from build123d import *

# Parameters (mm, degrees)
SKETCH1_W           = 30
SKETCH1_H           = 30
SKETCH1_W_2         = 26
SKETCH1_H_2         = 26
BOSS_EXTRUDE1_DEPTH = 248
SKETCH2_R           = 12
SKETCH2_R_2         = 10
BOSS_EXTRUDE2_DEPTH = 5


with BuildPart() as part:
    # Sketch1 → Boss-Extrude1 (new body)
    with BuildSketch(Plane.XY):
        Rectangle(SKETCH1_W, SKETCH1_H)
        Rectangle(SKETCH1_W_2, SKETCH1_H_2, mode=Mode.SUBTRACT)
    extrude(amount=BOSS_EXTRUDE1_DEPTH)

    # Sketch2 → Boss-Extrude2 (add)
    # profile 1 of 2: a face of its own
    with BuildSketch(Plane(origin=(15, 0, 0), x_dir=(0, 0, -1), z_dir=(1, 0, 0))):
        with Locations(Location((-19.522331238, 0, 0), (0, 0, 180))):
            Circle(SKETCH2_R)
        with Locations((-19.522331238, 0)):
            Circle(SKETCH2_R_2, mode=Mode.SUBTRACT)
    # profile 2 of 2: a face of its own
    with BuildSketch(Plane(origin=(15, 0, 0), x_dir=(0, 0, -1), z_dir=(1, 0, 0))):
        with Locations(Location((-228.477668762, 0, 0), (0, 0, 180))):
            Circle(SKETCH2_R)
        with Locations(Location((-228.477668762, 0, 0), (0, 0, 180))):
            Circle(SKETCH2_R_2, mode=Mode.SUBTRACT)
    extrude(amount=BOSS_EXTRUDE2_DEPTH)


solid = part.part
Source: CAD feature listing. Evaluate the final solid. Frame: model axes, mm. A direction names the side the tool comes from. Give positions to 0.01 mm unless a question says otherwise; leave off trailing zeros. Write each loop counter-clockwise with the first axis right and the second up, starting at its lowest first coordinate (ties: lowest second). Pieces come first, ordered by that corner, then holes. Notation, with made-up numbers: M 15,78.25 L 74,78.25 A28 ccw 74,104.25 Z; hole C 85,41.5 d11. An arc over 180 degrees is marked long. Return JSON: item names as keys, results as strings. Group by question number.
1) Cut plane C-C, the plane z = 154.5. Output: boundary loops of the cut face in (x, y), plus the area to 3 significant figures.
2) Cut plane D-D, the plane z = 227. Output: boundary loops of the cut face in (x, y).
3) Pin query (flat end, axial travel): P1, Ø1.5, axis at y = -4, z = 118.5, coming from the +X side. Return the tip coordinate at first contact, or that it passes through.
4) Pull-direction query (Y, two-part tool) for faces 4 (the face through (-13, 0, 122)), 5 (the face through (15, 0, 122)), 6 (the face through (0, -15, 122)); classes: pulls with the +Y half, pulls with the -Y half, needs draft (parallel to the pull), parting line crosses it, or undercut.
5) Set-up query: faces 1 (the face through (15, 0, 228)), 2 (the face through (-14, 0, 248)), 3 (the face through (13, 0, 122)). Return all of +Z, -Z, +X, -X, +Y, -Y with unobstructed straight access to the full face (end or side cutting, diameter ignored); none if empty.
6) Cut plane A-A, the plane y = 0. Output: boundary loops of the cut face in (x, z).
7) Material intervals for line 1 along Y through (x, z) = (-9.5, 192.5); line 2 along X through (y, z) = (11.5, 17.5), sorted ascending. Write a range as [from, to].
8) Cut plane B-B, the plane x = -7. Output: boundary loops of the cut face in (y, z), plus the area to 3 significant figures.
Recorded:
{
 "1": {"outline": "M -15,-15 L 15,-15 L 15,15 L -15,15 Z; hole M -13,-13 L 13,-13 L 13,13 L -13,13 Z", "area": "224 mm²"},
 "2": {"outline": "M -15,-15 L 15,-15 L 15,-11.91 L 20,-11.91 L 20,-9.89 L 15,-9.89 L 15,9.89 L 20,9.89 L 20,11.91 L 15,11.91 L 15,15 L -15,15 Z; hole M -13,-13 L 13,-13 L 13,13 L -13,13 Z"},
 "3": {"P1": "stops at x = 15"},
 "4": {"face 4": "undercut", "face 5": "needs draft", "face 6": "pulls with the -Y half"},
 "5": {"face 1": "+X", "face 2": "+Z, +X, -X, +Y, -Y", "face 3": "+Z, -Z"},
 "6": {"outline": "M -15,0 L -13,0 L -13,248 L -15,248 Z; M 13,0 L 15,0 L 15,7.52 L 20,7.52 L 20,9.52 L 15,9.52 L 15,29.52 L 20,29.52 L 20,31.52 L 15,31.52 L 15,216.48 L 20,216.48 L 20,218.48 L 15,218.48 L 15,238.48 L 20,238.48 L 20,240.48 L 15,240.48 L 15,248 L 13,248 Z"},
 "7": {"line 1": "y = [-15, -13], [13, 15]", "line 2": "x = [-15, -13], [13, 20]"},
 "8": {"outline": "M -15,0 L -13,0 L -13,248 L -15,248 Z; M 13,0 L 15,0 L 15,248 L 13,248 Z", "area": "992 mm²"}
}
